For this review, take the finished solid that the model builds, in its own axes (mm). Face numbers are marked on the shaded views. A direction names the side the tool comes from. Give positions to 0.01 mm unless a question says otherwise; leave off trailing zeros. Order: outer loops, then holes, each group sorted by start corner. A loop starts at its lowest first (then second) coordinate and runs counter-clockwise, first axis right, second up. Notation, with made-up numbers: (-19.75, -34) - (11.25, -34) arc R22 cw to (11.25, -26) - close; hole circle Ø10 at (51.5, -15.75). An arc over 180 degrees is marked (long way). One line per item, written item: value.
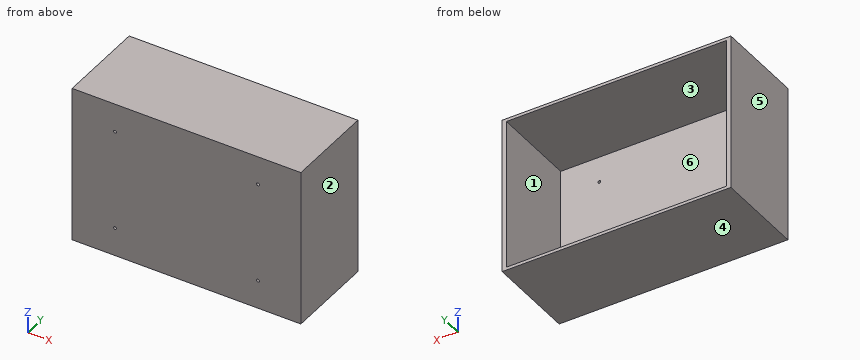
```python
from build123d import *

# Parameters (mm, degrees)
SKETCH_1_W          = 160
SKETCH_1_H          = 110
EXTRUDE_1_DEPTH     = 3
SKETCH_2_W          = 160
SKETCH_2_H          = 110
SKETCH_2_W_2        = 154
SKETCH_2_H_2        = 105.875
EXTRUDE_2_DEPTH     = 60
SKETCH_3_R          = 1
CUT_EXTRUDE_1_DEPTH = 10


with BuildPart() as part:
    # 草图1 → 凸台-拉伸1 (new body)
    with BuildSketch(Plane(origin=(0, 0, 0), x_dir=(1, 0, 0), z_dir=(0, 1, 0))):
        Rectangle(SKETCH_1_W, SKETCH_1_H)
    extrude(amount=EXTRUDE_1_DEPTH)

    # 草图2 → 凸台-拉伸2 (add)
    with BuildSketch(Plane(origin=(0, 3, 0), x_dir=(1, 0, 0), z_dir=(0, 1, 0))):
        Rectangle(SKETCH_2_W, SKETCH_2_H)
        Rectangle(SKETCH_2_W_2, SKETCH_2_H_2, mode=Mode.SUBTRACT)
    extrude(amount=EXTRUDE_2_DEPTH)

    # 草图3 → 切除-拉伸1 (cut)
    with BuildSketch(Plane(origin=(0, 3, 0), x_dir=(1, 0, 0), z_dir=(0, 1, 0))):
        with Locations((-50, 35)):
            Circle(SKETCH_3_R)
        with Locations((50, 35)):
            Circle(SKETCH_3_R)
        with Locations((50, -35)):
            Circle(SKETCH_3_R)
        with Locations((-50, -35)):
            Circle(SKETCH_3_R)
    extrude(amount=-CUT_EXTRUDE_1_DEPTH, mode=Mode.SUBTRACT)


solid = part.part
```
(1) Draft analysis for pull direction Z (two halves, no side actions). For the marked faces 1, 2, 3 and 4, state which applies: pulls with the +Z half, pulls with the -Z half, needs draft (parallel to the pull), parting line crosses it, or undercut.
Answers below:
face 1: undercut
face 2: needs draft
face 3: undercut
face 4: pulls with the -Z half
(2) Take a section at C-C (z = -0.5). Write out the cut boundary in (x, y), then the cut area to 3 significant figures.
Answers below:
outline: (-80, 0) - (80, 0) - (80, 63) - (77, 63) - (77, 3) - (-77, 3) - (-77, 63) - (-80, 63) - close
area: 840 mm^2
(3) For P1, Ø8, axis at x = -61.5, z = 15.5, coming from the +Y side; P2, Ø1.6, axis at x = 50, z = -35, coming from the -Y side, all flat-tipped, find the tip position at first contact; note any pin that passes through.
Answers below:
P1: stops at y = 3
P2: passes through
(4) Take a section at B-B (x = 6). Write out the cut boundary in (y, z).
Answers below:
outline: (0, -55) - (63, -55) - (63, -52.94) - (3, -52.94) - (3, 52.94) - (63, 52.94) - (63, 55) - (0, 55) - close
(5) Machinability: for the marked faces 5 and 6, which of the approach directions +Z, -Z, +X, -X, +Y, -Y give a long, thin tool a straight path to every point of the face, cutting with its end or side? Answer none if there is none.
Answers below:
face 5: +Z, -Z, -X, +Y, -Y
face 6: +Y
(6) Take a section at A-A (y = 12.5). Write out the cut boundary in (x, z).
Answers below:
outline: (-80, -55) - (80, -55) - (80, 55) - (-80, 55) - close; hole (-77, -52.94) - (77, -52.94) - (77, 52.94) - (-77, 52.94) - close
(7) Wall thickness on line 1 (Z direction, x = -50, y = 2); line 2 (Z direction, x = 55.5, y = 27); line 3 (X direction, y = 2.4, z = -35): over which ranges is each line inside the solid? List them lowest first. Write a range as from..to.
Answers below:
line 1: z = -55..-36, -34..34, 36..55
line 2: z = -55..-52.94, 52.94..55
line 3: x = -80..-51, -49..49, 51..80
